The model under review builds one solid part; all positions refer to its coordinate system, in mm. Face numbers are marked on the shaded views. A direction names the side the tool comes from. Coordinates: 2 decimals unless noted, no trailing zeros. Write each loop counter-clockwise with the first axis right and the second up, starting at its lowest first coordinate (ties: lowest second). Pieces come first, ordered by that corner, then holes. Notation, with made-up numbers: (-31, 70.5) - (-14, 70.5) arc R24 ccw to (-14, 92.5) - close; hole circle Ø11 at (-12.75, 26.25). An arc over 180 degrees is marked (long way). Return JSON: item names as keys, results as strings. Group by question number.
(1) We need section C-C on z = 22.5. State the section outline as (x, y) points, then the cut area to 3 significant figures.
(2) To check wall thickness, follow L1, parallel to Z at x = -6.5, y = 10; L2, parallel to Y at x = 27.5, z = 44.5; L3, parallel to Z at x = -6.5, y = -22. State the ranges of each line that lie inside material, in increasing order. Write a range as from..to.
(3) For pin 1 Ø11 at (x, z) = (-3, 127.5) entering from -Y; pin 2 Ø8 at (x, z) = (7.5, 82.5) entering from +Y; pin 3 Ø8 at (y, z) = (21.5, 15.5) entering from -X, all flat-tipped, find the tip position at first contact; note any pin that passes through.
(4) Tool access review of the marked faces 1, 2, 3 and 4: name each direction out of +Z, -Z, +X, -X, +Y, -Y from which nothing blocks a thin tool from reaching the whole face with its end or side.
(5) We need section D-D on x = 0. State the section outline as (y, z) points, then the cut area to 3 significant figures.
(6) Draft analysis for pull direction Z (two halves, no side actions). For the marked faces 5, 6, 7 and 8, state which applies: released by +Z, released by -Z, zero draft, split by the parting line, or undercut.
(7) We need section B-B on x = 10. State the section outline as (y, z) points.
(8) We need section A-A on y = -34.5. State the section outline as (x, z) points, then the cut area to 3 significant figures.
```python
from build123d import *

# Parameters (mm, degrees)
EXTRUDE_1_DEPTH     = 120
CUT_EXTRUDE_1_REACH = 132
SKETCH_3_W          = 14
SKETCH_3_H          = 80
SKETCH_4_W          = 60
SKETCH_4_H          = 7
EXTRUDE_3_DEPTH     = 10
SKETCH_5_W          = 14
SKETCH_5_H          = 12
CUT_EXTRUDE_2_DEPTH = 3
CUT_EXTRUDE_START   = -48
CUT_EXTRUDE_3_DEPTH = 14


with BuildPart() as part:
    # Эскиз1 → Бобышка-Вытянуть1 (new body)
    with BuildSketch(Plane.XY):
        Polygon((7, 7), (7, 33), (14, 33), (14, 40), (0, 40), (0, 0), (30, 0), (30, 7), (23, 7), align=None)
    extrude_1 = extrude(amount=EXTRUDE_1_DEPTH)

    # Вырез-Вытянуть1: up to this face of the body (flat: up to its plane)
    cut_extrude_1_end = Plane(part.part.faces().sort_by_distance((18.5, 7, 60))[0])
    # Эскиз3 → Вырез-Вытянуть1 (cut, up to the picked face)
    with BuildSketch(Plane(origin=(0, 40, 0), x_dir=(1, 0, 0), z_dir=(0, 1, 0)), mode=Mode.PRIVATE) as cut_extrude_1_sk1:
        with Locations((7, -80)):
            Rectangle(SKETCH_3_W, SKETCH_3_H)
    cut_extrude_1_tool1 = split(extrude(cut_extrude_1_sk1.sketch, amount=-CUT_EXTRUDE_1_REACH, mode=Mode.PRIVATE), bisect_by=cut_extrude_1_end, keep=Keep.BOTH, mode=Mode.PRIVATE)
    cut_extrude_1 = cut_extrude_1_tool1.solids().sort_by(Axis((7, 40, 80), (0, -1, 0)))[0]
    add(cut_extrude_1, mode=Mode.SUBTRACT)

    # Зеркальное отражение1: Бобышка-Вытянуть1, Вырез-Вытянуть1 across plane
    add(extrude_1.mirror(Plane(origin=(0, 0, 120), x_dir=(0, 0, 1), z_dir=(-1, 0, 0))))
    add(cut_extrude_1.mirror(Plane(origin=(0, 0, 120), x_dir=(0, 0, 1), z_dir=(-1, 0, 0))), mode=Mode.SUBTRACT)

    # Эскиз4 → Бобышка-Вытянуть3 (add)
    with BuildSketch(Plane.XY.offset(120)):
        Polygon((-30, 0), (-30, -41.5), (-15, -41.5), (-15, -26.5), (15, -26.5), (15, -41.5), (30, -41.5), (30, 0), align=None)
        Polygon((-30, 48.5), (-30, 7), (30, 7), (30, 48.5), (12.5, 48.5), (12.5, 23.5), (-12.5, 23.5), (-12.5, 48.5), align=None)
        with Locations((0, 3.5)):
            Rectangle(SKETCH_4_W, SKETCH_4_H)
    extrude(amount=EXTRUDE_3_DEPTH)

    # Эскиз5 → Вырез-Вытянуть2 (cut)
    with BuildSketch(Plane(origin=(0, 7, 0), x_dir=(1, 0, 0), z_dir=(0, 1, 0))):
        with Locations((23, -94)):
            Rectangle(SKETCH_5_W, SKETCH_5_H)
    extrude(amount=-CUT_EXTRUDE_2_DEPTH, mode=Mode.SUBTRACT)

    # Эскиз6 → Вырез-Вытянуть3 (cut)
    with BuildSketch(Plane(origin=(0, 0, 0), x_dir=(-1, 0, 0), z_dir=(0, 0, -1)).offset(CUT_EXTRUDE_START)):
        Polygon((30, 0), (17, 7), (30, 7), align=None)
    extrude(amount=-CUT_EXTRUDE_3_DEPTH, mode=Mode.SUBTRACT)


solid = part.part
```
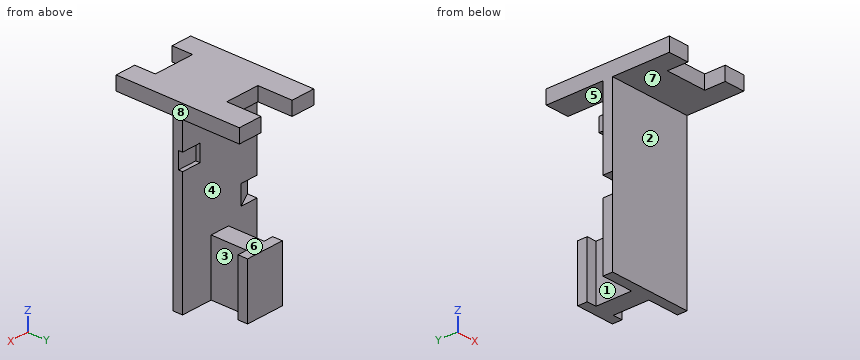
Ans:
{
 "1": {"outline": "(-30, 0) - (30, 0) - (30, 7) - (7, 7) - (7, 33) - (14, 33) - (14, 40) - (-14, 40) - (-14, 33) - (-7, 33) - (-7, 7) - (-30, 7) - close", "area": "980 mm²"},
 "2": {"L1": "0..40, 120..130", "L2": "0..7", "L3": "120..130"},
 "3": {"pin 1": "y = -26.5", "pin 2": "y = 7", "pin 3": "x = -7"},
 "4": {"face 1": "-Z, -X", "face 2": "-Z, +X, -X, -Y", "face 3": "-Z, +X", "face 4": "none"},
 "5": {"outline": "(-26.5, 120) - (0, 120) - (0, 0) - (40, 0) - (40, 40) - (7, 40) - (7, 120) - (23.5, 120) - (23.5, 130) - (-26.5, 130) - close", "area": "2,660 mm²"},
 "6": {"face 5": "undercut", "face 6": "undercut", "face 7": "released by -Z", "face 8": "zero draft"},
 "7": {"outline": "(-26.5, 120) - (0, 120) - (0, 0) - (7, 0) - (7, 120) - (23.5, 120) - (23.5, 130) - (-26.5, 130) - close; (33, 0) - (40, 0) - (40, 40) - (33, 40) - close"},
 "8": {"outline": "(-30, 120) - (-15, 120) - (-15, 130) - (-30, 130) - close; (15, 120) - (30, 120) - (30, 130) - (15, 130) - close", "area": "300 mm²"}
}
